Can you work these out from the model? Positions are in its coordinate system, mm. A direction names the side the tool comes from. Coordinates: 2 decimals unless noted, no trailing zeros. Order: outer loops, then holes, each group sorted by start corner. A loop starts at its lowest first (then second) coordinate and runs counter-clockwise, first axis right, second up. Notation, with made-up numbers: (5.25, 49) -> (62.25, 49) arc R30 cw to (62.25, 84) -> close; hole circle Ø2 at (28.5, -35). An arc over 180 degrees is marked (long way). Write item = value, one per line. Start each with the question number.
Autodesk Inventor part; units mm, degrees
ref_plane "YZ Plane" through (0, 0, 0) normal (1, 0, 0) x (0, 1, 0)
ref_plane "XZ Plane" through (0, 0, 0) normal (0, 1, 0) x (-1, 0, 0)
ref_plane "XY Plane" through (0, 0, 0) normal (0, 0, 1) x (1, 0, 0)
sketch "Эскиз1" plane through (0, 0, 0) normal (0, 0, 1) x (1, 0, 0)
  line L0 (0, 0) -> (19.6, 0)
  line L1 (19.6, 0) -> (19.6, 17.5)
  line L2 (19.6, 17.5) -> (0, 17.5)
  line L3 (0, 17.5) -> (0, 0)
  line L4 (0, 0) -> (0, 10.7)
  line L5 (0, 10.7) -> (19.6, 10.7)
  line L6 (19.6, 17.5) -> (17, 17.5)
  line L7 (19.6, 17.5) -> (19.6, 14.9)
  line L8 (19.6, 14.9) -> (17, 17.5)
  line L9 (0, 17.5) -> (2.6, 17.5)
  line L10 (0, 17.5) -> (0, 14.9)
  line L11 (0, 14.9) -> (2.6, 17.5)
  dimension "d0" = 19.6
  dimension "d1" = 17.5
  dimension "d2" = 10.7
  dimension "d3" = 2.6
  dimension "d4" = 2.6
  dimension "d5" = 2.6
  dimension "d6" = 2.6
extrude "Выдавливание1" add sketch "Эскиз1" along normal blind 1.6 contours L3 L5 L1 L0 | L3 L11 L2 L8 L1 L5
sketch "Эскиз2" plane through (0, 0, 1.6) normal (0, 0, 1) x (1, 0, 0)
  line L0 (2.6, 17.5) -> (0, 14.9)
  line L1 (19.6, 0) -> (19.6, 14.9)
  line L2 (0, 14.9) -> (19.6, 14.9)
  line L3 (19.6, 14.9) -> (9.8, 14.9)
  line L4 (17, 17.5) -> (2.6, 17.5)
  line L5 (9.8, 17.5) -> (9.8, 14.6)
  circle A0 centre (9.8, 14.6) radius 1.925
  point P0 (0, 0)
  dimension "d9" = 2.9
  dimension "d10" = 3.85
extrude "Выдавливание2" cut sketch "Эскиз2" against normal blind 1.6 contours A0 L5 L2 | L2 A0 | A0 L2 L5
sketch "Эскиз3" plane through (0, 0, 1.6) normal (0, 0, 1) x (1, 0, 0)
  line L0 (0, 14.9) -> (0, 0)
  line L1 (0, 0) -> (0, 10.3)
  line L2 (0, 0) -> (19.6, 0)
  line L3 (19.6, 0) -> (19.6, 10.3)
  line L4 (19.6, 0) -> (19.6, 14.9)
  line L5 (19.6, 10.3) -> (0, 10.3)
  dimension "d13" = 10.3
  dimension "d14" = 10.3
extrude "Выдавливание3" add sketch "Эскиз3" along normal blind 3.4
chamfer "Фаска1" distance 0.1 angle 45 1 edges at (9.8, 10.3, 5)
chamfer "Фаска2" distance 0.1 angle 45 16 edges at (19.6, 5.1, 5) (0, 5.1, 5) (9.8, 17.5, 1.6) (18.3, 16.2, 1.6) (19.6, 12.6, 1.6) (0, 12.6, 1.6) (1.3, 16.2, 1.6) (19.6, 14.9, 0.8) (17, 17.5, 0.8) (7.875, 14.6, 1.6) (7.875, 14.6, 0) (9.8, 17.5, 0) (18.3, 16.2, 0) (19.6, 7.45, 0) (19.6, 10.3, 3.25) (0, 10.3, 3.25)
chamfer "Фаска3" distance 0.2 angle 45 1 edges at (9.75, 0, 0)
chamfer "Фаска4" distance 0.2 angle 45 3 edges at (19.6, 0, 2.55) (0, 0, 2.55) (9.8, 0, 5)
chamfer "Фаска5" distance 0.1 angle 45 4 edges at (0, 7.55, 0) (1.25, 16.15, 0) (2.6, 17.5, 0.8) (0, 14.9, 0.75)
sketch "Эскиз4" plane through (0.2, 0, 4.8) normal (0, -1, 0) x (1, 0, 0)
  line L0 (0, -4.6) -> (0, 0)
  line L1 (19.2, 0) -> (19.2, -4.6)
  line L2 (0, 0) -> (19.2, 0)
  line L3 (19.2, 0) -> (19.2, -3.6)
  line L4 (19.2, -3.6) -> (0, -3.6)
  line L5 (0, -3.6) -> (0, 0)
  line L6 (-0.15, 0.15) -> (0, 0)
  line L7 (9.6, -1.8) -> (0, -1.8)
  line L8 (9.6, -1.8) -> (19.2, -1.8)
  line L9 (0, 0) -> (19.2, 0)
  line L10 (0, -3.6) -> (19.2, 0)
  line L11 (0, 0) -> (19.2, -3.6)
  line L12 (9.6, -1.8) -> (9.6, 0)
  line L13 (9.6, 0) -> (0, -3.6)
  line L14 (0, 0) -> (9.6, -3.6)
  line L15 (9.6, -3.6) -> (19.2, 0)
  line L16 (9.6, 0) -> (19.2, -3.6)
  line L17 (4.8, -1.8) -> (4.8, 0)
  line L18 (4.8, 0) -> (0, -3.6)
  line L19 (0, 0) -> (4.8, -3.6)
  line L20 (4.8, -3.6) -> (9.6, 0)
  line L21 (4.8, 0) -> (9.6, -3.6)
  line L22 (14.4, -1.8) -> (14.4, 0)
  line L23 (14.4, 0) -> (9.6, -3.6)
  line L24 (9.6, 0) -> (14.4, -3.6)
  line L25 (14.4, -3.6) -> (19.2, 0)
  line L26 (14.4, 0) -> (19.2, -3.6)
  line L27 (16.8, -1.8) -> (16.8, 0)
  line L28 (19.2, 0) -> (16.8, -3.6)
  line L29 (16.8, 0) -> (19.2, -3.6)
  line L30 (16.8, 0) -> (14.4, -3.6)
  line L31 (14.4, 0) -> (16.8, -3.6)
  line L32 (12, -1.8) -> (12, 0)
  line L33 (14.4, 0) -> (12, -3.6)
  line L34 (12, 0) -> (14.4, -3.6)
  line L35 (12, 0) -> (9.6, -3.6)
  line L36 (9.6, 0) -> (12, -3.6)
  line L37 (9.6, 0) -> (7.2, -3.6)
  line L38 (7.2, 0) -> (9.6, -3.6)
  line L39 (7.2, 0) -> (4.8, -3.6)
  line L40 (4.8, 0) -> (7.2, -3.6)
  line L41 (2.4, -1.8) -> (2.4, 0)
  line L42 (4.8, 0) -> (2.4, -3.6)
  line L43 (2.4, 0) -> (4.8, -3.6)
  line L44 (2.4, 0) -> (0, -3.6)
  line L45 (0, 0) -> (2.4, -3.6)
  circle A0 centre (1.2, -1.8) radius 0.35
  circle A1 centre (2.4, -1.8) radius 0.35
  circle A2 centre (3.6, -1.8) radius 0.35
  circle A3 centre (4.8, -1.8) radius 0.35
  circle A4 centre (6, -1.8) radius 0.35
  circle A5 centre (7.2, -1.8) radius 0.35
  circle A6 centre (8.4, -1.8) radius 0.35
  circle A7 centre (9.6, -1.8) radius 0.35
  circle A8 centre (10.8, -1.8) radius 0.35
  circle A9 centre (12, -1.8) radius 0.35
  circle A10 centre (13.2, -1.8) radius 0.35
  circle A11 centre (14.4, -1.8) radius 0.35
  circle A12 centre (15.6, -1.8) radius 0.35
  circle A13 centre (16.8, -1.8) radius 0.35
  circle A14 centre (18, -1.8) radius 0.35
  point P0 (-0.2, -4.8)
  dimension "d32" = 3.6
  dimension "d33" = 0.7
  dimension "d34" = 0.7
  dimension "d35" = 0.7
  dimension "d36" = 0.7
  dimension "d37" = 0.7
  dimension "d38" = 0.7
  dimension "d39" = 0.7
  dimension "d40" = 0.7
  dimension "d41" = 0.7
  dimension "d42" = 0.7
  dimension "d43" = 0.7
  dimension "d44" = 0.7
  dimension "d45" = 0.7
  dimension "d46" = 0.7
  dimension "d47" = 0.7
extrude "Выдавливание4" add sketch "Эскиз4" along normal blind 3 contours A0 L7 L44 | L44 L45 A0 | A0 L45 L7 | A1 L7 L18 | L18 L19 A1 | L45 L7 A0 | L44 A0 L7 | L45 A0 L44 | L19 L7 A1 | A2 L7 L42 | L42 L43 A2 | L18 A1 L7 | L41 A1 L18 | L7 A1 L19 | L19 A1 L41 | A5 L7 L20 | L20 L21 A5 | A4 L39 L40 | L40 L7 A4 | A3 L7 L13 | L13 L14 A3 | L43 L7 A2 | L42 A2 L7 | L43 A2 L42 | L7 A2 L43 | A8 L11 L35 | L35 L11 L36 A8 | A6 L37 L10 L38 | L38 L10 A6 | A6 L7 L37 L10 | L10 L37 A6 | L21 L7 A5 | L14 L7 A3 | A4 L7 L39 | L20 A5 L7 | L21 A5 L20 | L7 A5 L21 | L39 A4 L7 | L40 A4 L39 | L7 A4 L40 | L13 A3 L7 | L17 A3 L13 | L7 A3 L14 | L14 A3 L17 | L36 L11 A8 | L35 L36 L11 | L11 A8 L8 L35 | L38 L7 A6 L10 | L10 L37 L38 | A6 L11 L38 L7 | A7 L10 L12 | L12 L11 A7 | A8 L35 L10 L36 | L36 L10 A8 | A6 L11 L37 | L37 L11 L38 A6 | A6 L38 L11 | A9 L23 L24 | L24 L8 A9 | A10 L8 L33 | L33 L34 A10 | L11 L36 L8 A8 | A9 L8 L23 | L35 L10 A8 L8 | L36 L10 L35 | L8 A8 L10 L36 | A7 L10 L11 | L11 L8 A7 | L37 L11 A6 L7 | L38 L11 L37 | A7 L7 L10 | L10 A7 L8 | L7 A7 L11 | A8 L10 L35 | A11 L8 L15 | L15 L16 A11 | L34 L8 A10 | L23 A9 L8 | L32 A9 L23 | L8 A9 L24 | L24 A9 L32 | L33 A10 L8 | L34 A10 L33 | L8 A10 L34 | A14 L28 L29 | L29 L8 A14 | A13 L8 L25 | L25 L26 A13 | A12 L30 L31 | L31 L8 A12 | L16 L8 A11 | A12 L8 L30 | L15 A11 L8 | L22 A11 L15 | L8 A11 L16 | L16 A11 L22 | L8 L28 A14 | L26 L8 A13 | A14 L8 L28 | L29 A14 L28 | L8 A14 L29 | L25 A13 L8 | L27 A13 L25 | L8 A13 L26 | L26 A13 L27 | L30 A12 L8 | L31 A12 L30 | L8 A12 L31
sketch "Эскиз5" plane through (1.4, -3, 3) normal (0, -1, 0) x (1, 0, 0)
  point P0 (-1.4, -3)
properties part number "l298n"
(1) If I drill on L1, parallel to Y at x = 9.8, z = 0.55 (3 decimals); L2, parallel to X at y = 14.6, z = 0.8 (3 decimals); L3, parallel to Z at x = 5, y = 16.5, over which ranges is the centre line in solid material (lowest first)? Write a range as from..to.
(2) Imagine slicing it at C-C (z = 1.2). Write out the boundary of the cut face in (x, y) (3 decimals), plus the area to 3 significant figures.
(3) Thinking about a two-plate mould opening in X: for faces 3 (the face through (19.6, 6, 2)), 4 (the face through (10, 10.3, 3)), 5 (the face through (1.3, 16.2, 0.8)), 6 (the face through (10.835, 16.223, 0.81)), which applies, +X half, -X half, draft (parallel to the pull), parting line (faces both ways), or undercut?
(4) For P1, Ø1.6, axis at x = 11, z = 2.5, coming from the +Y side; P2, Ø3, axis at x = 17.5, y = 14, coming from the +Z side; P3, Ø2.5, axis at x = 9.8, y = 14.6, coming from the +Z side, each with a flat end and sliding along its axis, tell me the tip position at first contact or that it passes through.
(5) For faces 1 (the face through (10, 12, 1.6)), 2 (the face through (18.3, 16.2, 0.8)), which set-ups out of +Z, -Z, +X, -X, +Y, -Y let a thin tool reach every point of the face, with its end or its side?
(6) Imagine slicing it at A-A (x = 9.8). Write out the boundary of the cut face in (y, z) (3 decimals), plus the area to 3 significant figures.
(7) Imagine slicing it at D-D (x = 5). Write out the boundary of the cut face in (y, z), plus the area to 3 significant figures.
(8) Imagine slicing it at B-B (y = -0.5). Count the separate pieces of the cut face and the enclosed holes in it, plus the area to 3 significant figures.
Result set:
q1.L1 = 0..12.675, 16.525..17.5
q1.L2 = 0..7.875, 11.725..19.6
q1.L3 = 0..1.6
q2.outline = (0, 0.2) -> (0.2, 0) -> (19.4, 0) -> (19.6, 0.2) -> (19.6, 14.8) -> (19.529, 14.971) -> (17.071, 17.429) -> (16.9, 17.5) -> (2.7, 17.5) -> (2.529, 17.429) -> (0.071, 14.971) -> (0, 14.8) -> close; hole circle Ø3.85 at (9.8, 14.6)
q2.area = 325 mm2
q3.face_3 = +X half
q3.face_4 = draft
q3.face_5 = -X half
q3.face_6 = undercut
q4.P1 = 10.3
q4.P2 = 1.6
q4.P3 = through
q5.face_1 = +Z, +X, -X, +Y
q5.face_2 = +Z, -Z, +X, +Y
q6.outline = (-3, 2.65) -> (0, 2.65) -> (0, 0.2) -> (0.2, 0) -> (12.575, 0) -> (12.675, 0.1) -> (12.675, 1.5) -> (12.575, 1.6) -> (10.3, 1.6) -> (10.3, 4.9) -> (10.2, 5) -> (0.2, 5) -> (0, 4.8) -> (0, 3.35) -> (-3, 3.35) -> close; (16.525, 0.1) -> (16.625, 0) -> (17.4, 0) -> (17.5, 0.1) -> (17.5, 1.5) -> (17.4, 1.6) -> (16.625, 1.6) -> (16.525, 1.5) -> close
q6.area = 58.9 mm2
q7.outline = (-3, 2.65) -> (0, 2.65) -> (0, 0.2) -> (0.2, 0) -> (17.4, 0) -> (17.5, 0.1) -> (17.5, 1.5) -> (17.4, 1.6) -> (10.3, 1.6) -> (10.3, 4.9) -> (10.2, 5) -> (0.2, 5) -> (0, 4.8) -> (0, 3.35) -> (-3, 3.35) -> close
q7.area = 65.1 mm2
q8.separate_pieces = 15
q8.enclosed_holes = 0
q8.area = 5.77 mm2
